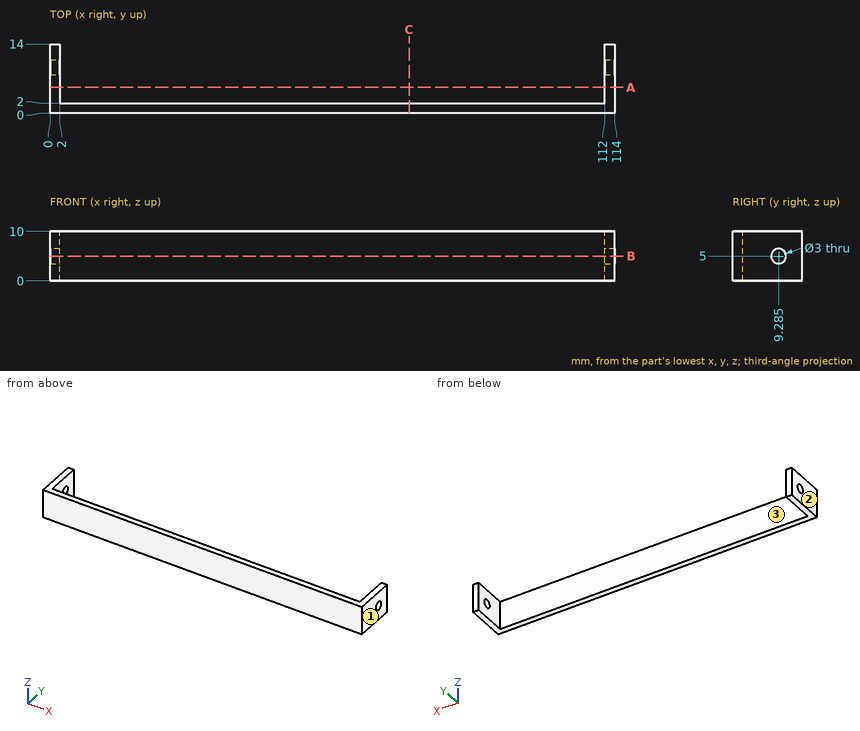
The figure shows three views and two pictorial views of one solid part (mm, origin at its lowest corner). Answer the questions. Coordinates: 2 decimals unless noted, no trailing zeros. Order: outer loops, then holes, each group sorted by start corner. A loop starts at its lowest first (then second) coordinate and runs counter-clockwise, first axis right, second up.
Q1. Consider line 1 (Y direction, x = 112.4, z = 5) (3 decimals); line 2 (X direction, y = 4, z = 7.75); line 3 (Y direction, x = 69.5, z = 6.25). Determine where each line is inside the solid, lowest interval first.
Q2. A cutting plane is placed at B-B, the plane z = 5. Write down the section's boundary in (x, y) (3 decimals), and give its area (3 significant figures).
Q3. A cutting plane is placed at C-C, the plane x = 72.5. Write down the section's boundary in (y, z).
Q4. A cutting plane is placed at A-A, the plane y = 5.25. Write down the section's boundary in (x, z).
Q5. Given P1, Ø5, axis at x = 80.5, z = 6, coming from the +Y side; P2, Ø3, axis at x = 79.5, z = 8.5, coming from the -Y side, each flat-ended and moving along its own axis, determine where each tip first touches the part or whether it passes through.
Q6. For a pull along X with two mould halves and no side action, classify the marked faces 1, 2 and 3 as pulls with the +X half, pulls with the -X half, needs draft (parallel to the pull), parting line crosses it, or undercut.
Answers follow:
1. line 1: y = 0 to 7.785, 10.785 to 14
1. line 2: x = 0 to 2, 112 to 114
1. line 3: y = 0 to 2
2. outline: (0, 0) - (114, 0) - (114, 7.785) - (112, 7.785) - (112, 2) - (2, 2) - (2, 7.785) - (0, 7.785) - close; (0, 10.785) - (2, 10.785) - (2, 14) - (0, 14) - close; (112, 10.785) - (114, 10.785) - (114, 14) - (112, 14) - close
2. area: 264 mm2
3. outline: (0, 0) - (2, 0) - (2, 10) - (0, 10) - close
4. outline: (0, 0) - (2, 0) - (2, 10) - (0, 10) - close; (112, 0) - (114, 0) - (114, 10) - (112, 10) - close
5. P1: stops at y = 2
5. P2: stops at y = 0
6. face 1: pulls with the +X half
6. face 2: pulls with the -X half
6. face 3: undercut
